```python
from build123d import *

# Parameters (mm, degrees)
SKETCH1_W           = 15
SKETCH1_H           = 18.5
SKETCH1_R           = 1.25
BOSS_EXTRUDE1_DEPTH = 2
SKETCH2_W           = 8.5
SKETCH2_H           = 3.5
BOSS_EXTRUDE2_DEPTH = 4
CHAMFER1_SIZE       = 3
CHAMFER1_SIZE2      = 12


with BuildPart() as part:
    # Sketch1 → Boss-Extrude1 (new body)
    with BuildSketch(Plane(origin=(0, 0, 0), x_dir=(1, 0, 0), z_dir=(0, 1, 0))):
        with Locations((7.5, 9.25)):
            Rectangle(SKETCH1_W, SKETCH1_H)
        with Locations(Location((2.5, 16, 0), (0, 0, 270))):
            Circle(SKETCH1_R, mode=Mode.SUBTRACT)
        with Locations(Location((12.5, 16, 0), (0, 0, 90))):
            Circle(SKETCH1_R, mode=Mode.SUBTRACT)
    extrude(amount=BOSS_EXTRUDE1_DEPTH)

    # Sketch2 → Boss-Extrude2 (add)
    with BuildSketch(Plane(origin=(0, 2, 0), x_dir=(1, 0, 0), z_dir=(0, 1, 0))):
        with Locations((7.5, 1.75)):
            Rectangle(SKETCH2_W, SKETCH2_H)
        Polygon((3.25, 9.25), (11.75, 9.25), (9.1, 21.5), (9.6, 21.5), (9.6, 24.5), (5.4, 24.5), (5.4, 21.5), (5.9, 21.5), align=None)
    extrude(amount=BOSS_EXTRUDE2_DEPTH)

    # Chamfer1
    chamfer1_edges = [part.edges().sort_by_distance(p)[0] for p in [
        (7.5, 6, -9.25),
    ]]
    chamfer1_side = [part.faces().sort_by_distance(p)[0] for p in [
        (7.5, 4, -9.25),
    ]]
    chamfer(chamfer1_edges, length=CHAMFER1_SIZE, length2=CHAMFER1_SIZE2, reference=chamfer1_side[0])


solid = part.part
```
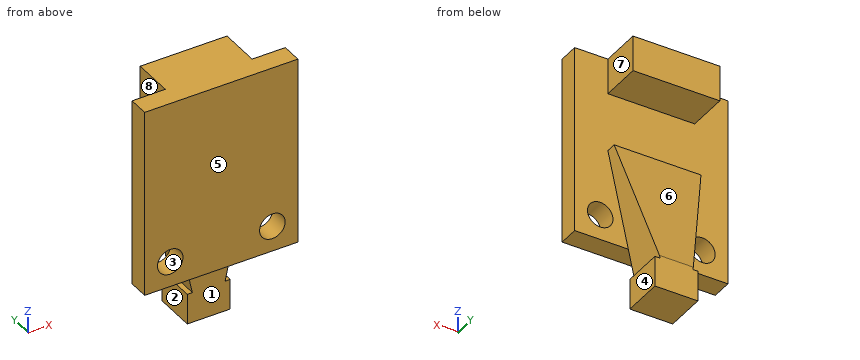
Model file for the job. Use its own axes, mm. Face numbers are marked on the shaded views. A direction names the side the tool comes from. Give positions to 0.01 mm unless a question says otherwise; leave off trailing zeros. Write each loop counter-clockwise with the first axis right and the second up, starting at its lowest first coordinate (ties: lowest second). Pieces come first, ordered by that corner, then holes. Notation, with made-up numbers: (35.5, 64.5) -> (76.5, 64.5) arc R26 cw to (76.5, 100.5) -> close; hole circle Ø9 at (-11.5, 87). An arc over 180 degrees is marked (long way). Use CSV: the item, a comma, the result in double quotes. Start each with the question number.
1) Cut at A-A on x = 1.5. List the corners of the cut face in (y, z).
2) Two-plate mould, pull along X, no slides. Class the marked faces 1, 2 and 3: released by +X, released by -X, zero draft, split by the parting line, or undercut.
3) Pin check, flat tips, straight feed: P1, Ø2, axis at x = 7, z = -23, coming from the -Y side; P2, Ø3.5, axis at y = 4, z = -23, coming from the -X side; P3, Ø3, axis at x = 12.5, z = -16, coming from the +Y side; P4, Ø1.6, axis at x = 6.5, y = 1.5, coming from the -Z side. Stop position of each tip, or through.
4) Cut at B-B on y = 2.5. List the corners of the cut face in (x, z), plus the area to 3 significant figures.
5) Cut at D-D on x = 11. List the corners of the cut face in (y, z).
6) Cut at C-C on z = -16. List the corners of the cut face in (x, y), plus the area to 3 significant figures.
7) Tool access for the marked faces 4, 5, 6, 7 and 8: list every direction of +Z, -Z, +X, -X, +Y, -Y with a clear straight run to the whole face (end or side of a thin tool).
8) Drill centre lines: L1, parallel to X at y = 1.4, z = -16; L2, parallel to Z at x = 12.5, y = 0.95; L3, parallel to Y at x = 1.25, z = -13.75. Where is each one in solid material? Low to high.
Final values:
1,outline,"(0, -18.5) -> (2, -18.5) -> (2, -16.75) -> (0, -16.75) -> close; (0, -15.25) -> (2, -15.25) -> (2, 0) -> (0, 0) -> close"
2,face 1,"zero draft"
2,face 2,"released by -X"
2,face 3,"undercut"
3,P1,"stops at y = 2"
3,P2,"stops at x = 5.4"
3,P3,"stops at y = 2"
3,P4,"stops at z = -24.5"
4,outline,"(3.25, -9.25) -> (5.9, -21.5) -> (5.4, -21.5) -> (5.4, -24.5) -> (9.6, -24.5) -> (9.6, -21.5) -> (9.1, -21.5) -> (11.75, -9.25) -> close; (3.25, -3.5) -> (11.75, -3.5) -> (11.75, 0) -> (3.25, 0) -> close"
4,area,"114 mm2"
5,outline,"(0, -18.5) -> (2, -18.5) -> (2, -12.72) -> (3.87, -12.72) -> (3, -9.25) -> (2, -9.25) -> (2, -3.5) -> (6, -3.5) -> (6, 0) -> (0, 0) -> close"
6,outline,"(0, 0) -> (1.25, 0) -> (1.25, 2) -> (0, 2) -> close; (3.75, 0) -> (11.25, 0) -> (11.25, 2) -> (10.29, 2) -> (10.29, 4.69) -> (4.71, 4.69) -> (4.71, 2) -> (3.75, 2) -> close; (13.75, 0) -> (15, 0) -> (15, 2) -> (13.75, 2) -> close"
6,area,"35.0 mm2"
7,face 4,"-Z, +X, +Y, -Y"
7,face 5,"+Z, -Z, +X, -X, -Y"
7,face 6,"+X, -X, +Y"
7,face 7,"+Z, -Z, +X, +Y"
7,face 8,"+Z, -Z, -X, +Y"
8,L1,"x = 0 to 1.25, 3.75 to 11.25, 13.75 to 15"
8,L2,"z = -18.5 to -17.25, -14.75 to 0"
8,L3,"y = 0 to 2"
